CAD build for the part. Positions are in the model's coordinates, mm. A direction names the side the tool comes from. Give positions to 0.01 mm unless a question says otherwise; leave off trailing zeros. Write each loop counter-clockwise with the first axis right and the second up, starting at its lowest first coordinate (ties: lowest second). Pieces come first, ordered by that corner, then holes. Notation, with made-up numbers: (79, -37) -> (130, -37) arc R37 cw to (130, 1) -> close; hole circle Ø9 at (76, -30.5). An arc over 180 degrees is marked (long way). Answer as a JSON object with one key per item and string values.
```python
from build123d import *

# Parameters (mm, degrees)
SKETCH7_W                = 45
SKETCH7_H                = 45
SKETCH7_W_2              = 2.024682368
SKETCH7_H_2              = 6.385975888
SKETCH7_R                = 2
SKETCH7_R_2              = 1.875
BOSS_EXTRUDE5_DEPTH      = 5
SKETCH7_3_W              = 45
SKETCH7_3_H              = 2
BOSS_EXTRUDE6_DEPTH      = 40
BOSS_EXTRUDE7_DEPTH      = 5
SKETCH7_4_W              = 45
SKETCH7_4_H              = 8
BOSS_EXTRUDE8_DEPTH      = 40
SKETCH11_R               = 2.375
CUT_EXTRUDE16_DEPTH      = 1
CUT_EXTRUDE16_DEPTH_BACK = 56
SKETCH7_14_R             = 11
CUT_EXTRUDE17_DEPTH      = 1


with BuildPart() as part:
    # Sketch7 → Boss-Extrude5 (new body)
    with BuildSketch(Plane(origin=(0, 0, 0), x_dir=(1, 0, 0), z_dir=(0, 1, 0))):
        with Locations((5.831933892, -118.050969126)):
            Rectangle(SKETCH7_W, SKETCH7_H)
        with Locations((-12.180407292, -119.050969126)):
            Rectangle(SKETCH7_W_2, SKETCH7_H_2, mode=Mode.SUBTRACT)
        with Locations((5.831933892, -136.550969126)):
            Circle(SKETCH7_R, mode=Mode.SUBTRACT)
        with Locations((5.831933892, -101.550969126)):
            Circle(SKETCH7_R_2, mode=Mode.SUBTRACT)
    extrude(amount=BOSS_EXTRUDE5_DEPTH)

    # Sketch7_3 → Boss-Extrude6 (add)
    with BuildSketch(Plane(origin=(0, 0, 0), x_dir=(1, 0, 0), z_dir=(0, 1, 0))):
        with Locations((5.831933892, -141.550969126)):
            Rectangle(SKETCH7_3_W, SKETCH7_3_H)
    extrude(amount=BOSS_EXTRUDE6_DEPTH)

    # Sketch8 → Boss-Extrude7 (add)
    with BuildSketch(Plane.ZY.offset(16.668066108)):
        Polygon((140.550969126, 11), (140.550969126, 5), (121.550969126, 5), (140.550969126, 19), align=None)
    boss_extrude7 = extrude(amount=-BOSS_EXTRUDE7_DEPTH)

    # Mirror2: Boss-Extrude7 across plane
    add(boss_extrude7.mirror(Plane.ZY.offset(-5.831933892)))

    # Sketch7_4 → Boss-Extrude8 (add)
    with BuildSketch(Plane(origin=(0, 0, 0), x_dir=(1, 0, 0), z_dir=(0, 1, 0))):
        with Locations((5.831933892, -146.550969126)):
            Rectangle(SKETCH7_4_W, SKETCH7_4_H)
    extrude(amount=BOSS_EXTRUDE8_DEPTH)

    # Sketch11 → Cut-Extrude16 (cut, two sides)
    with BuildSketch(Plane.XY.offset(150.550969126)) as cut_extrude16_sk:
        with Locations((-10.168066108, 27)):
            Circle(SKETCH11_R)
        with Locations((21.831933892, 27)):
            Circle(SKETCH11_R)
    extrude(amount=CUT_EXTRUDE16_DEPTH, mode=Mode.SUBTRACT)
    extrude(cut_extrude16_sk.sketch, amount=-CUT_EXTRUDE16_DEPTH_BACK, mode=Mode.SUBTRACT)

    # Sketch7_14 → Cut-Extrude17 (cut)
    with BuildSketch(Plane(origin=(0, 0, 0), x_dir=(1, 0, 0), z_dir=(0, 1, 0))):
        with Locations((12.831933892, -119.050969126)):
            Circle(SKETCH7_14_R)
    extrude(amount=CUT_EXTRUDE17_DEPTH, mode=Mode.SUBTRACT)


solid = part.part
```
1) Slice it at D-D (y = 32). List the corners of the cut face in (x, z).
Model answer:
{"outline": "(-16.67, 140.55) -> (28.33, 140.55) -> (28.33, 150.55) -> (-16.67, 150.55) -> close"}
2) 3-axis set-ups, long thin cutter, end or side, ignore diameter. For faces 4 (the flat face through (-16.668, 15, 136)), 5 (the cylindrical face through (24.026, 26.09, 145.621)), 6 (the flat face through (-12, 2, 122.244)), 7 (the flat face through (6, 5, 118)), 8 (the flat face through (-12, 2, 115.858)): which of +Z, -Z, +X, -X, +Y, -Y reach the whole face in a straight line?
Model answer:
{"face 4": "+Z, -Z, -X, +Y, -Y", "face 5": "+Z, -Z", "face 6": "-Y", "face 7": "-Z, +Y", "face 8": "+Y, -Y"}
3) Slice it at C-C (z = 145.5). List the corners of the cut face in (x, y) (3 decimals).
Model answer:
{"outline": "(-16.668, 0) -> (28.332, 0) -> (28.332, 40) -> (-16.668, 40) -> close; hole circle Ø4.75 at (-10.168, 27); hole circle Ø4.75 at (21.832, 27)"}
4) Pin check, flat tips, straight feed: pin 1 (2 mm diameter, centred on x = 9.5, z = 113, fed in from +Y); pin 2 (1 mm diameter, centred on x = -1, y = 15.5, fed in from -Z). Stop position of each tip, or through.
Model answer:
{"pin 1": "stops at y = 5", "pin 2": "stops at z = 140.55"}
5) Slice it at A-A (y = 27). List the corners of the cut face in (x, z), then the cut area to 3 significant figures.
Model answer:
{"outline": "(-16.67, 140.55) -> (-12.54, 140.55) -> (-12.54, 150.55) -> (-16.67, 150.55) -> close; (-7.79, 140.55) -> (19.46, 140.55) -> (19.46, 150.55) -> (-7.79, 150.55) -> close; (24.21, 140.55) -> (28.33, 140.55) -> (28.33, 150.55) -> (24.21, 150.55) -> close", "area": "355 mm2"}
6) Mould opens along Z. For faces 1 (the flat face through (-11.168, 2, 119)), 2 (the flat face through (28.332, 15, 136)), 3 (the flat face through (6, 20, 150.551)) say: released by +Z, released by -Z, zero draft, split by the parting line, or undercut.
Model answer:
{"face 1": "undercut", "face 2": "zero draft", "face 3": "released by +Z"}
7) Slice it at B-B (x = 25). List the corners of the cut face in (y, z), then the cut area to 3 significant figures.
Model answer:
{"outline": "(0, 95.55) -> (5, 95.55) -> (5, 121.55) -> (19, 140.55) -> (40, 140.55) -> (40, 150.55) -> (0, 150.55) -> close", "area": "758 mm2"}
8) Wall check: probe 1 along Y at (x, z) = (-4, 132); probe 2 along Z at (x, y) = (-0.5, 6); probe 3 along Y at (x, z) = (20.5, 121.5). Give the ranges that are in metal, low to high.
Model answer:
{"probe 1": "y = 0 to 5", "probe 2": "z = 140.55 to 150.55", "probe 3": "y = 1 to 5"}
